from build123d import *

# Parameters (mm, degrees)
SCHIZZO1_R                   = 3.5
ESTRUSIONE_ESTRUSIONE1_DEPTH = 18
SCHIZZO2_R                   = 2.5
ESTRUSIONE_ESTRUSIONE2_DEPTH = 8
ESTRUSIONE_ESTRUSIONE3_START = 8
SCHIZZO3_R                   = 2.5
ESTRUSIONE_ESTRUSIONE3_DEPTH = 8
SMUSSO1_SIZE                 = 0.5


with BuildPart() as part:
    # Schizzo1 → Estrusione-Estrusione1 (new, symmetric)
    with BuildSketch(Plane(origin=(0, 0, 0), x_dir=(0, 0, -1), z_dir=(1, 0, 0))):
        with Locations((-80, 0)):
            Circle(SCHIZZO1_R)
    extrude(amount=ESTRUSIONE_ESTRUSIONE1_DEPTH, both=True)

    # Schizzo2 → Estrusione-Estrusione2 (add)
    with BuildSketch(Plane(origin=(18, 0, 0), x_dir=(0, 0, -1), z_dir=(1, 0, 0))):
        with Locations((-80, 0)):
            Circle(SCHIZZO2_R)
    extrude(amount=ESTRUSIONE_ESTRUSIONE2_DEPTH)

    # Schizzo3 → Estrusione-Estrusione3 (add)
    with BuildSketch(Plane.ZY.offset(18).offset(ESTRUSIONE_ESTRUSIONE3_START)):
        with Locations(Location((80, 0, 0), (0, 0, 180))):
            Circle(SCHIZZO3_R)
    extrude(amount=-ESTRUSIONE_ESTRUSIONE3_DEPTH)

    # Smusso1
    smusso1_edges = [part.edges().sort_by_distance(p)[0] for p in [
        (-26, 0, 82.5),
        (26, 0, 82.5),
    ]]
    chamfer(smusso1_edges, length=SMUSSO1_SIZE)


solid = part.part
Read the model definition and answer for the solid it produces. Units are mm, in the model's axes. A direction names the side the tool comes from. Coordinates: 2 decimals unless noted, no trailing zeros. Loops run counter-clockwise (first coordinate to the right, second up) from the corner with the lowest first, then second, coordinate; pieces in that order, holes last. Notation, with made-up numbers: (15.25, 20) - (60.25, 20) arc R23 cw to (60.25, 40) - close; hole circle Ø5 at (-33.5, 84.25). An arc over 180 degrees is marked (long way). Answer in a Markdown table with one row per item.
Q1. Given P1, Ø3, axis at x = -13.5, y = -2, coming from the -Z side; P2, Ø1.5, axis at x = -4.5, z = 79, coming from the -Y side; P3, Ø1, axis at x = -20.5, y = -0.5, coming from the -Z side, each flat-ended and moving along its own axis, determine where each tip first touches the part or whether it passes through.
Here are the results:
| item | result |
|---|---|
| P1 | stops at z = 76.54 |
| P2 | stops at y = -3.49 |
| P3 | stops at z = 77.5 |
Q2. Find section B-B on x = 22. Write down the section's boundary in (y, z), plus the area to 3 significant figures.
Here are the results:
| item | result |
|---|---|
| outline | circle Ø5 at (0, 80) |
| area | 19.6 mm^2 |
Q3. Find section A-A on z = 80. Write down the section's boundary in (x, y), plus the area to 4 significant figures.
Here are the results:
| item | result |
|---|---|
| outline | (-26, -2) - (-25.5, -2.5) - (-18, -2.5) - (-18, -3.5) - (18, -3.5) - (18, -2.5) - (25.5, -2.5) - (26, -2) - (26, 2) - (25.5, 2.5) - (18, 2.5) - (18, 3.5) - (-18, 3.5) - (-18, 2.5) - (-25.5, 2.5) - (-26, 2) - close |
| area | 331.5 mm^2 |
Q4. Find section C-C on x = 16.5. Write down the section's boundary in (y, z).
Here are the results:
| item | result |
|---|---|
| outline | circle Ø7 at (0, 80) |
Q5. For faces 1 (the flat face through (26, 0, 80)), 2 (the flat face through (-18, -2, 78)), 3 (the cylindrical face through (21.7, 0.1, 82.5)), determine the directions among +Z, -Z, +X, -X, +Y, -Y from which every point of the face is accessible in a straight line to the end or side of a thin tool.
Here are the results:
| item | result |
|---|---|
| face 1 | +Z, -Z, +X, +Y, -Y |
| face 2 | -X |
| face 3 | +X |
Q6. Straight lines are drawn through the part: line 1 along X through (y, z) = (2.5, 81.75); line 2 along X through (y, z) = (0.5, 82); line 3 along Y through (x, z) = (14, 81). For each, find the intervals that lie inside material, in ascending order. Write a range as [from, to].
Here are the results:
| item | result |
|---|---|
| line 1 | x = [-18, 18] |
| line 2 | x = [-25.94, 25.94] |
| line 3 | y = [-3.35, 3.35] |
